Can you work these out from the model? Positions are in its coordinate system, mm. Face numbers are marked on the shaded views. A direction names the side the tool comes from. Coordinates: 2 decimals unless noted, no trailing zeros. Loops run counter-clockwise (first coordinate to the right, second up) from the corner with the lowest first, then second, coordinate; pieces in that order, holes last.
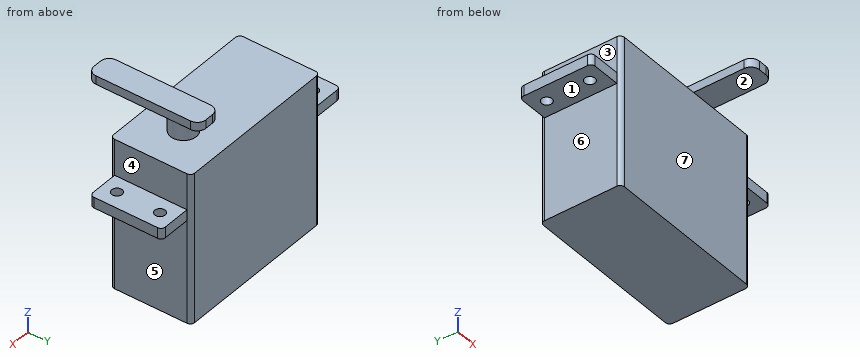
```python
from build123d import *

# Parameters (mm, degrees)
BOSS_EXTRUDE1_DEPTH = 34.9
BOSS_EXTRUDE2_DEPTH = 2.5
SKETCH3_R           = 1.2
CUT_EXTRUDE1_DEPTH  = 2.5
SKETCH4_R           = 3
BOSS_EXTRUDE3_DEPTH = 4
BOSS_EXTRUDE4_DEPTH = 2


with BuildPart() as part:
    # Sketch1 → Boss-Extrude1 (new body)
    with BuildSketch(Plane.XY):
        with BuildLine():
            Line((-18.3, -9.4), (18.3, -9.4))
            ThreePointArc((18.3, -9.4), (19.007106781, -9.107106781), (19.3, -8.4))
            Line((19.3, -8.4), (19.3, 8.4))
            ThreePointArc((19.3, 8.4), (19.007106781, 9.107106781), (18.3, 9.4))
            Line((18.3, 9.4), (-18.3, 9.4))
            ThreePointArc((-18.3, 9.4), (-19.007106781, 9.107106781), (-19.3, 8.4))
            Line((-19.3, 8.4), (-19.3, -8.4))
            ThreePointArc((-19.3, -8.4), (-19.007106781, -9.107106781), (-18.3, -9.4))
        make_face()
    extrude(amount=BOSS_EXTRUDE1_DEPTH)

    # Sketch2 → Boss-Extrude2 (add)
    with BuildSketch(Plane.XY.offset(24)):
        with BuildLine():
            Line((-25.8, -8.4), (25.8, -8.4))
            ThreePointArc((25.8, -8.4), (26.507106781, -8.107106781), (26.8, -7.4))
            Line((26.8, -7.4), (26.8, 7.4))
            ThreePointArc((26.8, 7.4), (26.507106781, 8.107106781), (25.8, 8.4))
            Line((25.8, 8.4), (-25.8, 8.4))
            ThreePointArc((-25.8, 8.4), (-26.507106781, 8.107106781), (-26.8, 7.4))
            Line((-26.8, 7.4), (-26.8, -7.4))
            ThreePointArc((-26.8, -7.4), (-26.507106781, -8.107106781), (-25.8, -8.4))
        make_face()
    extrude(amount=BOSS_EXTRUDE2_DEPTH)

    # Sketch3 → Cut-Extrude1 (cut)
    with BuildSketch(Plane.XY.offset(24)):
        with Locations((23, 5)):
            Circle(SKETCH3_R)
        with Locations((23, -5)):
            Circle(SKETCH3_R)
        with Locations((-23, 5)):
            Circle(SKETCH3_R)
        with Locations((-23, -5)):
            Circle(SKETCH3_R)
    extrude(amount=CUT_EXTRUDE1_DEPTH, mode=Mode.SUBTRACT)

    # Sketch4 → Boss-Extrude3 (add)
    with BuildSketch(Plane.XY.offset(34.9)):
        with Locations((9.5, 0)):
            Circle(SKETCH4_R)
    extrude(amount=BOSS_EXTRUDE3_DEPTH)

    # Sketch5 → Boss-Extrude4 (add)
    with BuildSketch(Plane.XY.offset(38.9)):
        with BuildLine():
            Line((8.5, -20), (10.5, -20))
            ThreePointArc((10.5, -20), (11.914213562, -19.414213562), (12.5, -18))
            Line((12.5, -18), (12.5, 4))
            ThreePointArc((12.5, 4), (11.914213562, 5.414213562), (10.5, 6))
            Line((10.5, 6), (8.5, 6))
            ThreePointArc((8.5, 6), (7.085786438, 5.414213562), (6.5, 4))
            Line((6.5, 4), (6.5, -18))
            ThreePointArc((6.5, -18), (7.085786438, -19.414213562), (8.5, -20))
        make_face()
    extrude(amount=BOSS_EXTRUDE4_DEPTH)


solid = part.part
```
(1) I want a section at C-C on x = 9.5. Write out the boundary of the cut face in (y, z).
Check values:
outline: (-20, 38.9) - (-3, 38.9) - (-3, 34.9) - (-9.4, 34.9) - (-9.4, 0) - (9.4, 0) - (9.4, 34.9) - (3, 34.9) - (3, 38.9) - (6, 38.9) - (6, 40.9) - (-20, 40.9) - close
(2) Which directions (+Z, -Z, +X, -X, +Y, -Y) give clear straight access to the entire face, cutting with the end or side of a thin tool? Please do the marked faces 4, 5, 6 and 7.
Check values:
face 4: +Z, +X, +Y, -Y
face 5: -Z, +X, +Y, -Y
face 6: -Z, -X, +Y, -Y
face 7: -Z, +X, -X, -Y
(3) I want a section at B-B on x = 23. Write out the boundary of the cut face in (y, z), then the cut area to 3 significant figures.
Check values:
outline: (-8.4, 24) - (-6.2, 24) - (-6.2, 26.5) - (-8.4, 26.5) - close; (-3.8, 24) - (3.8, 24) - (3.8, 26.5) - (-3.8, 26.5) - close; (6.2, 24) - (8.4, 24) - (8.4, 26.5) - (6.2, 26.5) - close
area: 30.0 mm2
(4) I want a section at D-D on z = 28.5. Write out the boundary of the cut face in (x, y), then the cut area to 3 significant figures.
Check values:
outline: (-19.3, -8.4) arc R1 ccw to (-18.3, -9.4) - (18.3, -9.4) arc R1 ccw to (19.3, -8.4) - (19.3, 8.4) arc R1 ccw to (18.3, 9.4) - (-18.3, 9.4) arc R1 ccw to (-19.3, 8.4) - close
area: 725 mm2
(5) I'm going to push flat-ended pins straight in: pin 1 (6 mm diameter, centred on y = 4, z = 4.5, fed in from +X); pin 2 (6 mm diameter, centred on x = 21.5, y = -0.5, fed in from +Z); pin 3 (8 mm diameter, centred on x = -15, z = 7, fed in from -Y); pin 4 (2 mm diameter, centred on x = 3.5, z = 36.5, fed in from -Y). Where does each tip first touch, or does it pass through?
Check values:
pin 1: stops at x = 19.3
pin 2: stops at z = 34.9
pin 3: stops at y = -9.4
pin 4: passes through
(6) If we mould it in two halves opening along Z, with no side actions, what happens to the marked faces 1, 2 and 3? For each: released by +Z, released by -Z, zero draft, split by the parting line, or undercut.
Check values:
face 1: released by -Z
face 2: undercut
face 3: zero draft
(7) If I drill on probe 1 along Y at (x, z) = (-23, 25); probe 2 along Y at (x, z) = (-4.5, 17); probe 3 along Z at (x, y) = (-12, 6.5), over which ranges is the centre line in solid material (lowest first)?
Check values:
probe 1: y = -8.4 to -6.2, -3.8 to 3.8, 6.2 to 8.4
probe 2: y = -9.4 to 9.4
probe 3: z = 0 to 34.9
(8) I want a section at A-A on y = -5. Write out the boundary of the cut face in (x, z), then the cut area to 3 significant figures.
Check values:
outline: (-26.8, 24) - (-24.2, 24) - (-24.2, 26.5) - (-26.8, 26.5) - close; (-21.8, 24) - (-19.3, 24) - (-19.3, 0) - (19.3, 0) - (19.3, 24) - (21.8, 24) - (21.8, 26.5) - (19.3, 26.5) - (19.3, 34.9) - (-19.3, 34.9) - (-19.3, 26.5) - (-21.8, 26.5) - close; (6.5, 38.9) - (12.5, 38.9) - (12.5, 40.9) - (6.5, 40.9) - close; (24.2, 24) - (26.8, 24) - (26.8, 26.5) - (24.2, 26.5) - close
area: 1,380 mm2
